CAD build for the part. Positions are in the model's coordinates, mm. Face numbers are marked on the shaded views. A direction names the side the tool comes from. Coordinates: 2 decimals unless noted, no trailing zeros. Write each loop counter-clockwise with the first axis right and the second up, starting at its lowest first coordinate (ties: lowest second). Pieces come first, ordered by that corner, then holes. Notation, with made-up numbers: M 59,-5.5 L 72,-5.5 A20 ccw 72,19.5 Z; hole C -24,-25 d10. An arc over 180 degrees is marked long. Put each result on its own line as item: value. Start each with the question number.
Autodesk Inventor part; units mm, degrees
ref_plane "Work Plane1" through (0, 0, 5) normal (0, 0, 1) x (1, 0, 0)
ref_plane "YZ Plane" through (0, 0, 0) normal (1, 0, 0) x (0, 1, 0)
ref_plane "XZ Plane" through (0, 0, 0) normal (0, 1, 0) x (-1, 0, 0)
sketch "Sketch1" plane through (0, 0, 0) normal (0, 0, 1) x (1, 0, 0)
  circle A0 centre (0, 0) radius 17.5
  circle A1 centre (0, 0) radius 25.5
  dimension "d0" = 35
  dimension "d1" = 8
extrude "Extrusion1" add sketch "Sketch1" along normal blind 10
ref_plane "Work Plane1" through (0, 0, 5) normal (0, 0, 1) x (1, 0, 0)
sketch "Sketch2" plane through (0, 0, 5) normal (0, 0, 1) x (1, 0, 0)
  circle A0 centre (0, 0) radius 25.5
  circle A1 centre (0, 0) radius 21.5
  dimension "d4" = 4
extrude "Extrusion2" cut sketch "Sketch2" along normal mid plane 5
sketch "Sketch3" plane through (0, 0, 10) normal (0, 0, 1) x (1, 0, 0)
  circle A0 centre (0, 0) radius 17.5 construction
  line L0 (0, 0) -> (0, 17.5) construction
  line L1 (0, 17.5) -> (0, 22.5)
  arc A1 (14.4627, 17.236) -> (0, 22.5) centre (0, 0) ccw
  arc A2 (11.2488, 13.4058) -> (0, 17.5) centre (0, 0) ccw
  line L2 (14.4627, 17.236) -> (11.2488, 13.4058)
  dimension "d7" = 5
  dimension "d8" = 40
extrude "Extrusion3" add sketch "Sketch3" along normal blind 5
pattern_circular "Circular Pattern1" count 4 over 360 about axis through (0, 0, 0) along (0, 0, 1) of "Extrusion3"
mirror "Mirror1" about plane through (0, 0, 5) normal (0, 0, 1) of "Extrusion3", "Circular Pattern1"
sketch "Sketch4" plane through (0, 0, 10) normal (0, 0, 1) x (1, 0, 0)
  arc A0 (17.5, 0) -> (11.2488, 13.4058) centre (0, 0) ccw
  arc A1 (11.2488, 13.4058) -> (0, 17.5) centre (0, 0) ccw
  arc A2 (0, 17.5) -> (-13.4058, 11.2488) centre (0, 0) ccw
  arc A3 (-13.4058, 11.2488) -> (-17.5, 0) centre (0, 0) ccw
  arc A4 (-17.5, 0) -> (-11.2488, -13.4058) centre (0, 0) ccw
  arc A5 (-11.2488, -13.4058) -> (0, -17.5) centre (0, 0) ccw
  arc A6 (0, -17.5) -> (13.4058, -11.2488) centre (0, 0) ccw
  arc A7 (13.4058, -11.2488) -> (17.5, 0) centre (0, 0) ccw
  line L0 (4.7625, -4.7625) -> (-4.7625, -4.7625)
  line L1 (-4.7625, -4.7625) -> (-4.7625, 4.7625)
  line L2 (-4.7625, 4.7625) -> (4.7625, 4.7625)
  line L3 (4.7625, 4.7625) -> (4.7625, -4.7625)
  line L4 (4.7625, -4.7625) -> (-4.7625, 4.7625) construction
  line L5 (-4.7625, -4.7625) -> (4.7625, 4.7625) construction
  arc A8 (0, 17.5) -> (-13.4058, 11.2488) centre (0, 0) ccw
  circle A9 centre (0, 0) radius 17.5
  dimension "d14" = 9.525
extrude "Extrusion4" add sketch "Sketch4" against normal up to surface (20 mm away) from surface at 5
properties part number "dog clutch"
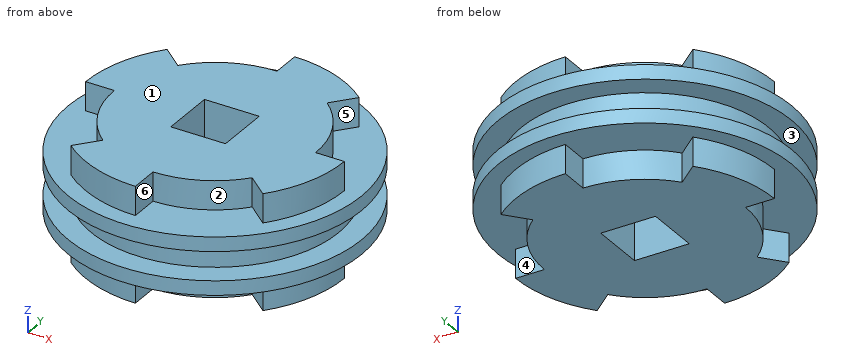
(1) Slice it at B-B, the plane y = -4. Write the cut outline in (x, z).
(2) Drill centre lines: line 1 (Z direction, x = -15.5, y = -15.5); line 2 (Z direction, x = -2, y = -21.5); line 3 (X direction, y = 3, z = 12). Where is each one in solid material? Low to high. Write a range as [from, to].
(3) Slice it at C-C, the plane x = 16. Write the cut outline in (y, z), then the cut area to 3 significant figures.
(4) Slice it at A-A, the plane z = 3.5. Write the cut outline in (x, y), then the cut area to 3 significant figures.
(5) Slice it at D-D, the plane y = 8. Write the cut outline in (x, z), then the cut area to 3 significant figures.
(6) Drop flat-ended pins along their axis: pin 1 (1.5 mm diameter, centred on x = 15, z = -2, fed in from +Y); pin 2 (2 mm diameter, centred on y = 20, z = 9.5, fed in from +X); pin 3 (5.5 mm diameter, centred on x = 21, z = -3, fed in from +Y). Give the stop position or say it passes through.
(7) Two-plate mould, pull along Z, no slides. Class the marked faces 1, 2 and 3: +Z half, -Z half, draft (parallel to the pull), parting line (faces both ways), or undercut.
(8) Which spindle directions (+Z, -Z, +X, -X, +Y, -Y) get a long thin tool onto all of the face, cutting with end or side? Do the marked faces 4, 5 and 6. Say none if no direction does.
Result set:
1. outline: M -25.18,0 L -17.04,0 L -17.04,-5 L -4.76,-5 L -4.76,15 L -17.04,15 L -17.04,10 L -25.18,10 L -25.18,7.5 L -21.12,7.5 L -21.12,2.5 L -25.18,2.5 Z; M 4.76,-5 L 22.14,-5 L 22.14,0 L 25.18,0 L 25.18,2.5 L 21.12,2.5 L 21.12,7.5 L 25.18,7.5 L 25.18,10 L 22.14,10 L 22.14,15 L 4.76,15 Z
2. line 1: z = [0, 2.5], [7.5, 10]
2. line 2: z = [-5, 2.5], [7.5, 15]
2. line 3: x = [-22.3, -4.76], [4.76, 17.24]
3. outline: M -19.86,0 L -13.43,0 L -13.43,-5 L 7.09,-5 L 7.09,0 L 19.86,0 L 19.86,2.5 L 14.36,2.5 L 14.36,7.5 L 19.86,7.5 L 19.86,10 L 7.09,10 L 7.09,15 L -13.43,15 L -13.43,10 L -19.86,10 L -19.86,7.5 L -14.36,7.5 L -14.36,2.5 L -19.86,2.5 Z
3. area: 547 mm^2
4. outline: C 0,0 d43; hole M -4.76,-4.76 L 4.76,-4.76 L 4.76,4.76 L -4.76,4.76 Z
4. area: 1,360 mm^2
5. outline: M -24.21,0 L -21.03,0 L -21.03,-5 L 15.56,-5 L 15.56,0 L 24.21,0 L 24.21,2.5 L 19.96,2.5 L 19.96,7.5 L 24.21,7.5 L 24.21,10 L 15.56,10 L 15.56,15 L -21.03,15 L -21.03,10 L -24.21,10 L -24.21,7.5 L -19.96,7.5 L -19.96,2.5 L -24.21,2.5 Z
5. area: 808 mm^2
6. pin 1: stops at y = 17.41
6. pin 2: stops at x = 17.01
6. pin 3: stops at y = 0
7. face 1: +Z half
7. face 2: draft
7. face 3: undercut
8. face 4: -Z, +X, +Y
8. face 5: +Z, +X
8. face 6: +Z, +X, -Y
